Autodesk Inventor part; units mm, degrees
ref_plane "YZ Plane" through (0, 0, 0) normal (1, 0, 0) x (0, 1, 0)
ref_plane "XZ Plane" through (0, 0, 0) normal (0, 1, 0) x (-1, 0, 0)
ref_plane "XY Plane" through (0, 0, 0) normal (0, 0, 1) x (1, 0, 0)
sketch "Sketch1" plane through (0, 0, 0) normal (0, 1, 0) x (-1, 0, 0)
  line L0 (-1.44, 25.5171) -> (-11.6, 25.5171)
  line L1 (-11.6, 25.5171) -> (-11.6, -73.5429)
  line L2 (-11.6, -73.5429) -> (-1.44, -73.5429)
  line L3 (-1.44, -73.5429) -> (-1.44, 25.5171)
  point P0 (0, 0)
  dimension "d0" = 99.06
  dimension "d1" = 10.16
extrude "Extrusion1" add sketch "Sketch1" along normal blind 101.6
sketch "Sketch2" plane through (0, 101.6, 0) normal (0, 1, 0) x (1, 0, 0)
  line L0 (1.44, -25.5171) -> (11.6, -25.5171)
  point P0 (0, 0)
  point P1 (6.5886, -19.1671)
  point P2 (6.5886, 6.2329)
  dimension "d4" = 0
  dimension "d5" = 6.35
  dimension "d6" = 25.4
hole "Hole1" at (6.5886, 101.6, 19.1671) at (6.5886, 101.6, -6.2329) direction (0, -1, 0) diameter 2.6416 end through all
sketch "Sketch3" plane through (11.6, 0, 25.5171) normal (1, 0, 0) x (0, 0, -1)
  line L0 (12.7, 88.9) -> (-33.0221, 88.9)
  line L1 (-33.0221, 88.9) -> (-33.0221, 24.13)
  line L2 (-33.0221, 24.13) -> (12.7, 24.13)
  line L3 (12.7, 24.13) -> (12.7, 88.9)
  line L4 (0, 101.6) -> (99.06, 101.6)
  line L5 (0, 0) -> (0, 101.6)
  point P0 (25.5171, 0)
  dimension "d15" = 12.7
  dimension "d16" = 64.77
  dimension "d19" = 12.7
extrude "Extrusion2" cut sketch "Sketch3" against normal blind 25.4
sketch "Sketch4" plane through (11.6, 0, 25.5171) normal (1, 0, 0) x (0, 0, -1)
  line L0 (12.7, 24.13) -> (44.45, 24.13)
  line L1 (44.45, 24.13) -> (44.45, 88.9)
  line L2 (44.45, 88.9) -> (12.7, 88.9)
  line L3 (12.7, 88.9) -> (12.7, 24.13)
  line L4 (0, 88.9) -> (12.7, 88.9)
  line L5 (12.7, 24.13) -> (0, 24.13)
  line L6 (12.7, 88.9) -> (12.7, 24.13)
  point P0 (25.5171, 0)
  dimension "d20" = 31.75
  dimension "d21" = 0
  dimension "d22" = 0
  dimension "d23" = 0
extrude "Extrusion3" cut sketch "Sketch4" against normal blind 25.4
sketch "Sketch5" plane through (0, 101.6, 0) normal (0, 1, 0) x (1, 0, 0)
  circle A0 centre (6.5886, 6.2329) radius 1.3208
  circle A1 centre (6.5886, -19.1671) radius 1.3208
  point P0 (0, 0)
hole "Hole2" at (6.5886, 101.6, 19.1671) at (6.5886, 101.6, -6.2329) direction (0, -1, 0) diameter 3.81 depth 15.24 tip angle 118.188
fillet "Fillet1" radius 3.175 1 edges at (11.6, 95.25, 25.5171)
fillet "Fillet2" radius 3.175 5 edges at (11.6, 12.065, 25.5171) (1.44, 12.065, 25.5171) (1.44, 95.25, 25.5171) (11.6, 50.8, -73.5429) (1.44, 50.8, -73.5429)
properties part number "GripperPlate"
Model file for the job. Use its own axes, mm. A direction names the side the tool comes from. Round coordinates to 2 decimals unless told otherwise and drop trailing zeros. Order: outer loops, then holes, each group sorted by start corner. A loop starts at its lowest first (then second) coordinate and runs counter-clockwise, first axis right, second up. Notation, with made-up numbers: (0, -32.75) -> (32, -32.75) arc R10 ccw to (32, -21.75) -> close; hole circle Ø2 at (55, -1). An arc over 180 degrees is marked (long way). Use one line per item in the form item = value.
Item 1: Cut at B-B, the plane y = 16. Write the cut outline in (x, z) (3 decimals), and give its area (3 significant figures).
Returned:
outline = (1.44, -70.368) arc R3.175 ccw to (4.615, -73.543) -> (8.425, -73.543) arc R3.175 ccw to (11.6, -70.368) -> (11.6, 22.342) arc R3.175 ccw to (8.425, 25.517) -> (4.615, 25.517) arc R3.175 ccw to (1.44, 22.342) -> close; hole circle Ø2.642 at (6.589, -6.233); hole circle Ø2.642 at (6.589, 19.167)
area = 987 mm^2
Item 2: Drill centre lines: line 1 (Y direction, x = 7.75, z = -4); line 2 (Z direction, x = 7.5, y = 12.5); line 3 (Z direction, x = 7, y = 21.5). Where is each one in solid material? Low to high.
Returned:
line_1 = 0 to 24.13, 88.9 to 101.6
line_2 = -73.54 to -7.19, -5.28 to 18.21, 20.12 to 25.52
line_3 = -73.54 to -7.49, -4.98 to 17.91, 20.42 to 25.52
Item 3: Flat gauge pin, fed straight in: pin 1 Ø5 at (x, y) = (10.5, 15.5) entering from +Z. Where does the tip first touch, or does it go through?
Returned:
pin_1 = 25.52
Item 4: Cut at A-A, the plane z = 16. Write the cut outline in (x, y), and give its area (3 significant figures).
Returned:
outline = (1.44, 0) -> (11.6, 0) -> (11.6, 24.13) -> (1.44, 24.13) -> close; (1.44, 88.9) -> (11.6, 88.9) -> (11.6, 101.6) -> (1.44, 101.6) -> close
area = 374 mm^2
Item 5: Pull direction Z, two halves, no side cores. Call faces 4 (the face through (7, 101.6, -23)), 5 (the face through (7.392, 11.896, -7.281)), 6 (the face through (2.345, 95.339, 24.562)), 7 (the face through (6.531, 11.896, 17.848)): released by +Z, released by -Z, zero draft, split by the parting line, or undercut.
Returned:
face_4 = zero draft
face_5 = undercut
face_6 = released by +Z
face_7 = undercut
Item 6: Tool access for faces 1 (the face through (6.505, 95.161, 17.264)), 2 (the face through (10.645, 12.234, 24.612)), 3 (the face through (7, 56, -18.933)): list every direction of +Z, -Z, +X, -X, +Y, -Y with a clear straight run to the whole face (end or side of a thin tool).
Returned:
face_1 = +Y
face_2 = +Z, +X, +Y, -Y
face_3 = +Z, +X, -X
Item 7: Cut at D-D, the plane x = 9.75. Write the cut outline in (y, z), and give its area (3 significant figures).
Returned:
outline = (0, -73.25) -> (101.6, -73.25) -> (101.6, 25.23) -> (88.9, 25.23) -> (88.9, -18.93) -> (24.13, -18.93) -> (24.13, 25.23) -> (0, 25.23) -> close
area = 7,150 mm^2
Item 8: Cut at C-C, the plane y = 70. Write the cut outline in (x, z) (3 decimals), and give its area (3 significant figures).
Returned:
outline = (1.44, -70.368) arc R3.175 ccw to (4.615, -73.543) -> (8.425, -73.543) arc R3.175 ccw to (11.6, -70.368) -> (11.6, -18.933) -> (1.44, -18.933) -> close
area = 551 mm^2
